Check sheet for the modelled part. Datum: model origin and axes. Units: mm. A direction names the side the tool comes from. Round coordinates to 2 decimals unless told otherwise and drop trailing zeros. Write each loop counter-clockwise with the first axis right and the second up, starting at its lowest first coordinate (ties: lowest second). Pieces come first, ordered by that corner, then holes. Notation, with made-up numbers: (64, 63) -> (72, 63) arc R19 ccw to (72, 93) -> close; hole circle Ø10 at (22.5, 86). An arc over 180 degrees is marked (long way). One line per item, written item: value. Start each with the question number.
```python
from build123d import *

# Parameters (mm, degrees)
EXTRUDE_1_DEPTH     = 6
SKETCH_2_R          = 3.5
CUT_EXTRUDE_1_DEPTH = 73.360210061
SKETCH_3_W          = 40
SKETCH_3_H          = 20
CUT_EXTRUDE_2_DEPTH = 121


with BuildPart() as part:
    # 草图1 → 凸台-拉伸1 (new body)
    with BuildSketch(Plane.XY):
        with BuildLine():
            Line((-52, -40), (52, -40))
            ThreePointArc((52, -40), (57.656854249, -37.656854249), (60, -32))
            Line((60, -32), (60, 32))
            ThreePointArc((60, 32), (57.656854249, 37.656854249), (52, 40))
            Line((52, 40), (-52, 40))
            ThreePointArc((-52, 40), (-57.656854249, 37.656854249), (-60, 32))
            Line((-60, 32), (-60, -32))
            ThreePointArc((-60, -32), (-57.656854249, -37.656854249), (-52, -40))
        make_face()
    extrude(amount=EXTRUDE_1_DEPTH)

    # 草图2 → 切除-拉伸1 (cut, through all)
    with BuildSketch(Plane.XY):
        with Locations((-48, -28)):
            Circle(SKETCH_2_R)
        with Locations((-48, 28)):
            Circle(SKETCH_2_R)
        with Locations((48, -28)):
            Circle(SKETCH_2_R)
        with Locations((48, 28)):
            Circle(SKETCH_2_R)
    extrude(amount=CUT_EXTRUDE_1_DEPTH, mode=Mode.SUBTRACT)

    # 草图3 → 切除-拉伸2 (cut, symmetric)
    with BuildSketch(Plane.XY):
        Rectangle(SKETCH_3_W, SKETCH_3_H)
    extrude(amount=CUT_EXTRUDE_2_DEPTH, both=True, mode=Mode.SUBTRACT)


solid = part.part
```
1. Cross-section at C-C (y = 28). Record the cut outline in (x, z).
2. Material ranges on probe 1 along X at (y, z) = (-28, 1.6); probe 2 along Y at (x, z) = (48, 1.5); probe 3 along Y at (x, z) = (-51, 5.55), recorded low to high.
3. Cross-section at B-B (x = 48). Record the cut outline in (y, z), plus the area to 3 significant figures.
4. Release check for a two-part mould opening along Y. For faces 1 (the face through (-57.594, 37.719, 2.958)), 2 (the face through (-1, 18, 6)), 3 (the face through (45.42, -25.635, 2.958)) record: +Y half, -Y half, draft (parallel to the pull), parting line (faces both ways), or undercut.
5. Cross-section at D-D (z = 4.8). Record the cut outline in (x, y).
6. Cross-section at A-A (x = 2). Record the cut outline in (y, z), plus the area to 3 significant figures.
7. Depth check by flat-ended pin: pin 1 Ø8 at (x, y) = (-48, 28) entering from +Z. Enter the tip coordinate at first touch or a pass-through.
8. Access from +Z, -Z, +X, -X, +Y, -Y to the whole of each face (thin tool, end or side, straight path). Record for faces 4 (the face through (0, -10, 3)), 5 (the face through (-1, -40, 3)).
Working result:
1. outline: (-60, 0) -> (-51.5, 0) -> (-51.5, 6) -> (-60, 6) -> close; (-44.5, 0) -> (44.5, 0) -> (44.5, 6) -> (-44.5, 6) -> close; (51.5, 0) -> (60, 0) -> (60, 6) -> (51.5, 6) -> close
2. probe 1: x = -60 to -51.5, -44.5 to 44.5, 51.5 to 60
2. probe 2: y = -40 to -31.5, -24.5 to 24.5, 31.5 to 40
2. probe 3: y = -40 to -29.8, -26.2 to 26.2, 29.8 to 40
3. outline: (-40, 0) -> (-31.5, 0) -> (-31.5, 6) -> (-40, 6) -> close; (-24.5, 0) -> (24.5, 0) -> (24.5, 6) -> (-24.5, 6) -> close; (31.5, 0) -> (40, 0) -> (40, 6) -> (31.5, 6) -> close
3. area: 396 mm^2
4. face 1: +Y half
4. face 2: draft
4. face 3: undercut
5. outline: (-60, -32) arc R8 ccw to (-52, -40) -> (52, -40) arc R8 ccw to (60, -32) -> (60, 32) arc R8 ccw to (52, 40) -> (-52, 40) arc R8 ccw to (-60, 32) -> close; hole circle Ø7 at (-48, -28); hole circle Ø7 at (-48, 28); hole (-20, -10) -> (20, -10) -> (20, 10) -> (-20, 10) -> close; hole circle Ø7 at (48, -28); hole circle Ø7 at (48, 28)
6. outline: (-40, 0) -> (-10, 0) -> (-10, 6) -> (-40, 6) -> close; (10, 0) -> (40, 0) -> (40, 6) -> (10, 6) -> close
6. area: 360 mm^2
7. pin 1: stops at z = 6
8. face 4: +Z, -Z
8. face 5: +Z, -Z, +X, -X, -Y
